The listing builds one solid part. Answer for the finished solid, in the listing's coordinates (mm). A direction names the side the tool comes from. Give positions to 0.01 mm unless a question says otherwise; leave off trailing zeros. Write each loop counter-clockwise with the first axis right and the second up, starting at its lowest first coordinate (ties: lowest second). Pieces come first, ordered by that corner, then holes.
```python
from build123d import *

# Parameters (mm, degrees)
ESQUISSE1_W      = 150
ESQUISSE1_H      = 250
EXTRUSION1_DEPTH = 150
ESQUISSE2_R      = 10
EXTRUSION2_DEPTH = 200
ESQUISSE3_W      = 80
ESQUISSE3_H      = 80
EXTRUSION3_DEPTH = 80


with BuildPart() as part:
    # Esquisse1 → Extrusion1 (new body)
    with BuildSketch(Plane(origin=(0, 0, 0), x_dir=(1, 0, 0), z_dir=(0, 1, 0))):
        with Locations((75, 125)):
            Rectangle(ESQUISSE1_W, ESQUISSE1_H)
    extrude(amount=EXTRUSION1_DEPTH)

    # Esquisse2 → Extrusion2 (add)
    with BuildSketch(Plane(origin=(0, 150, 0), x_dir=(1, 0, 0), z_dir=(0, 1, 0))):
        with Locations((75, 125)):
            Circle(ESQUISSE2_R)
    extrude(amount=EXTRUSION2_DEPTH)

    # Esquisse3 → Extrusion3 (add)
    with BuildSketch(Plane(origin=(0, 350, 0), x_dir=(1, 0, 0), z_dir=(0, 1, 0))):
        with Locations((75, 125)):
            Rectangle(ESQUISSE3_W, ESQUISSE3_H)
    extrude(amount=EXTRUSION3_DEPTH)


solid = part.part
```
Item 1: Which of the six approach directions +Z, -Z, +X, -X, +Y, -Y give full straight-line access (tool end or side, diameter ignored) to faces 5 (the face through (74, 389, -85)), 6 (the face through (35, 389, -124)), 7 (the face through (115, 389, -124)), 8 (the face through (74, 389, -165))?
Conclusion:
face 5: +Z, +X, -X, +Y
face 6: +Z, -Z, -X, +Y
face 7: +Z, -Z, +X, +Y
face 8: -Z, +X, -X, +Y
Item 2: A cutting plane is placed at C-C, the plane y = 283.5. Give the vertices of the cut face in (x, z).
Conclusion:
outline: circle Ø20 at (75, -125)
Item 3: Determine the mould class of faces 1 (the face through (74, 430, -126)), 2 (the face through (74, 74, 0)), 3 (the face through (66, 350, -117)), 4 (the face through (74, 0, -127)) for opening direction Y: pulls with the +Y half, pulls with the -Y half, needs draft (parallel to the pull), parting line crosses it, or undercut.
Conclusion:
face 1: pulls with the +Y half
face 2: needs draft
face 3: undercut
face 4: pulls with the -Y half
Item 4: Consider probe 1 along Y at (x, z) = (52, -156); probe 2 along Y at (x, z) = (76, -204.5); probe 3 along Z at (x, y) = (74.5, 230). Determine where each line is inside the solid, lowest interval first.
Conclusion:
probe 1: y = 0 to 150, 350 to 430
probe 2: y = 0 to 150
probe 3: z = -134.99 to -115.01
Item 5: A cutting plane is placed at A-A, the plane x = 92. Give the vertices of the cut face in (y, z), plus the area to 3 significant figures.
Conclusion:
outline: (0, -250) - (150, -250) - (150, 0) - (0, 0) - close; (350, -165) - (430, -165) - (430, -85) - (350, -85) - close
area: 43,900 mm2
Item 6: Each of these flat-tipped pins is pushed along its axis until it touches: P1, Ø6, axis at x = 72.5, z = -63.5, coming from the +Y side; P2, Ø4, axis at y = 332.5, z = -122.5, coming from the +X side; P3, Ø8, axis at x = 83, z = -195, coming from the -Y side; P4, Ø24, axis at x = 79, y = 396, coming from the +Z side. Where does it stop, or does it pass through?
Conclusion:
P1: stops at y = 150
P2: stops at x = 84.99
P3: stops at y = 0
P4: stops at z = -85
Item 7: A cutting plane is placed at D-D, the plane x = 11. Give the vertices of the cut face in (y, z), plus the area to 3 significant figures.
Conclusion:
outline: (0, -250) - (150, -250) - (150, 0) - (0, 0) - close
area: 37,500 mm2
Item 8: A cutting plane is placed at B-B, the plane z = -125. Give the vertices of the cut face in (x, y).
Conclusion:
outline: (0, 0) - (150, 0) - (150, 150) - (85, 150) - (85, 350) - (115, 350) - (115, 430) - (35, 430) - (35, 350) - (65, 350) - (65, 150) - (0, 150) - close
